from build123d import *

# Parameters (mm, degrees)
F0_R     = 30
F0_R_2   = 27.5
F1_DEPTH = 1100
F2_R     = 70
F3_DEPTH = 5
F4_R     = 30
F4_R_2   = 27.5
F5_DEPTH = 200


with BuildPart() as f1:
    # F0 (on Front) → F1 (new body, symmetric)
    with BuildSketch(Plane.XZ):
        Circle(F0_R)
        Circle(F0_R_2, mode=Mode.SUBTRACT)
    extrude(amount=F1_DEPTH, both=True)

    # F2 (on face) → F3 (join)
    with BuildSketch(Plane.XZ.offset(1100)):
        Circle(F2_R)
    extrude(amount=F3_DEPTH)

    # F4 (on face) → F5 (join)
    with BuildSketch(Plane.XZ.offset(1105)):
        Circle(F4_R)
        Circle(F4_R_2, mode=Mode.SUBTRACT)
    extrude(amount=F5_DEPTH)


solid = f1.part
Input: part model. Units: mm. Frame: model coordinates. A direction names the side the tool comes from. Coordinates: 2 decimals unless noted, no trailing zeros. Order: outer loops, then holes, each group sorted by start corner. A loop starts at its lowest first (then second) coordinate and runs counter-clockwise, first axis right, second up. Notation, with made-up numbers: M 23,39.5 L 56,39.5 A9 ccw 56,53.5 Z; hole C 79,45 d9. An arc over 180 degrees is marked long. Answer in a Markdown table with one row per item.
(1) Contact query for flat-ended pins moving along their axis: pin 1 Ø1.5 at (x, y) = (-11.5, -183.5) entering from -Z; pin 2 Ø5 at (x, y) = (12.5, 719.5) entering from -Z; pin 3 Ø1 at (x, z) = (-43, 49.5) entering from -Y. Output: stop coordinate, or through.
Numbers:
| item | result |
|---|---|
| pin 1 | stops at z = -28.01 |
| pin 2 | stops at z = -28.28 |
| pin 3 | stops at y = -1105 |
(2) Section query A-A, the plane x = 0. Output: boundary loops of the cut face in (y, z), plus the area to 3 significant figures.
Numbers:
| item | result |
|---|---|
| outline | M -1305,-30 L -1105,-30 L -1105,-70 L -1100,-70 L -1100,-30 L 1100,-30 L 1100,-27.5 L -1100,-27.5 L -1100,27.5 L 1100,27.5 L 1100,30 L -1100,30 L -1100,70 L -1105,70 L -1105,30 L -1305,30 L -1305,27.5 L -1105,27.5 L -1105,-27.5 L -1305,-27.5 Z |
| area | 12,700 mm^2 |
(3) Access query for faces 1 (the cylindrical face through (-5.961, 15.4, -26.846)), 2 (the flat face through (13.2, 1100, -24.3)), 3 (the cylindrical face through (-5.961, -1203.6, -26.846)). Directions: +Z, -Z, +X, -X, +Y, -Y. A direction counts if a zero-diameter tool reaches every point of the face in a straight line with its end or side. Return the directions, or none.
Numbers:
| item | result |
|---|---|
| face 1 | +Y |
| face 2 | +Z, -Z, +X, -X, +Y |
| face 3 | -Y |
(4) Section query B-B, the plane z = 0. Output: boundary loops of the cut face in (x, y).
Numbers:
| item | result |
|---|---|
| outline | M -70,-1105 L -30,-1105 L -30,-1305 L -27.5,-1305 L -27.5,-1105 L 27.5,-1105 L 27.5,-1305 L 30,-1305 L 30,-1105 L 70,-1105 L 70,-1100 L 30,-1100 L 30,1100 L 27.5,1100 L 27.5,-1100 L -27.5,-1100 L -27.5,1100 L -30,1100 L -30,-1100 L -70,-1100 Z |
(5) Draft query along Z for faces 4 (the flat face through (30, -1100, -15)), 5 (the cylindrical face through (-29.97, -15.4, 1.32)), 6 (the flat face through (0, -1100, 0)). Return one class per face: pulls with the +Z half, pulls with the -Z half, needs draft (parallel to the pull), parting line crosses it, or undercut.
Numbers:
| item | result |
|---|---|
| face 4 | needs draft |
| face 5 | parting line crosses it |
| face 6 | undercut |
(6) Material intervals for line 1 (Z direction, x = 0, y = -1217.5); line 2 (X direction, y = -957, z = 5); line 3 (Z direction, x = -3, y = 375), sorted ascending. Write a range as [from, to].
Numbers:
| item | result |
|---|---|
| line 1 | z = [-30, -27.5], [27.5, 30] |
| line 2 | x = [-29.58, -27.04], [27.04, 29.58] |
| line 3 | z = [-29.85, -27.34], [27.34, 29.85] |
(7) Section query C-C, the plane y = -1071.5. Output: boundary loops of the cut face in (x, z).
Numbers:
| item | result |
|---|---|
| outline | C 0,0 d60; hole C 0,0 d55 |
